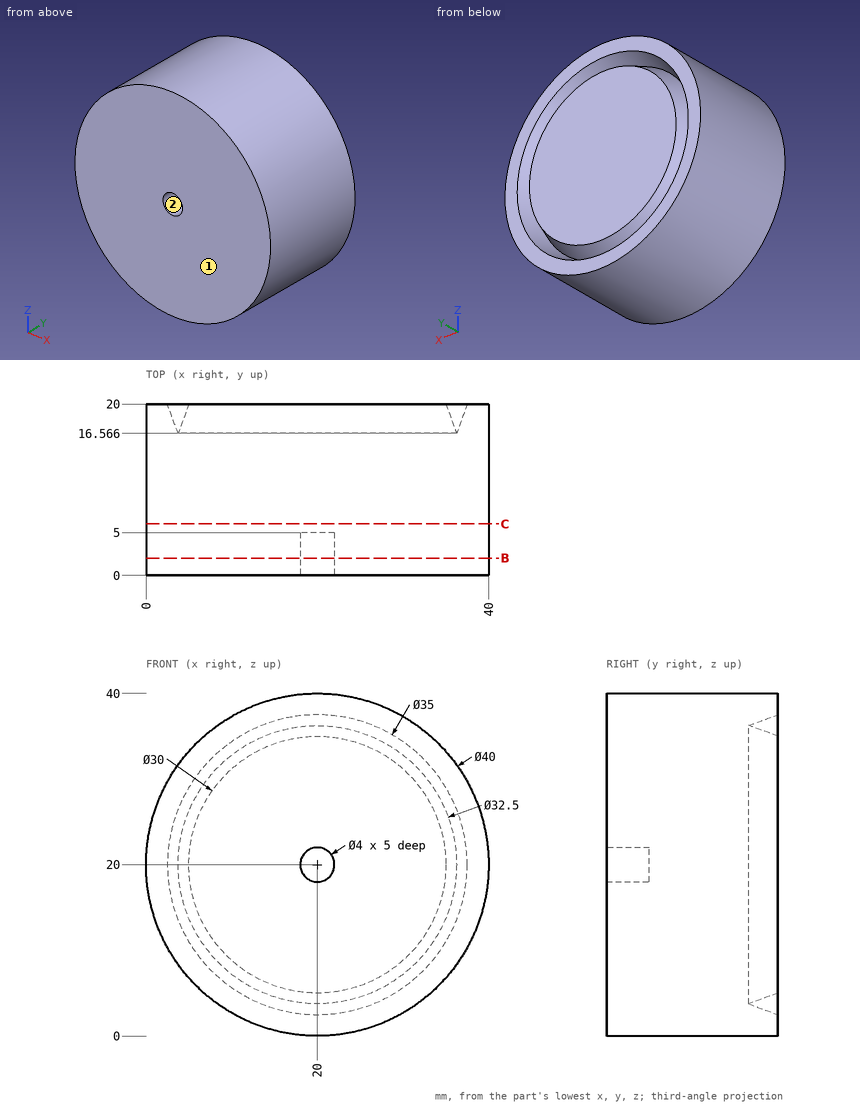
Design review of the part shown in the three views and the two pictorial views. Dimensions are in mm from the part's minimum x, y and z. A direction names the side the tool comes from. Round coordinates to 2 decimals unless told otherwise and drop trailing zeros. Loops run counter-clockwise (first coordinate to the right, second up) from the corner with the lowest first, then second, coordinate; pieces in that order, holes last. Notation, with made-up numbers: M 12,33 L 20,33 A25 ccw 20,65 Z; hole C 78.25,-13 d4. An arc over 180 degrees is marked long. Answer as a JSON object with one key per item and string values.
Item 1: Tool access review of the marked faces 1 and 2: name each direction out of +Z, -Z, +X, -X, +Y, -Y from which nothing blocks a thin tool from reaching the whole face with its end or side.
Check sheet entries:
{"face 1": "+Z, -Z, +X, -X, -Y", "face 2": "-Y"}
Item 2: For line 1 along X through (y, z) = (1.05, 20); line 2 along Z through (x, y) = (11, 19.25); line 3 along X through (y, z) = (17.25, 27.5) (1 decimal), list the stretches that pass through material, from the lowest coordinate up.
Check sheet entries:
{"line 1": "0 to 18, 22 to 40", "line 2": "2.14 to 5.31, 7.66 to 32.34, 34.69 to 37.86", "line 3": "1.5 to 5.3, 5.9 to 34.1, 34.7 to 38.5"}
Item 3: We need section C-C, the plane y = 6. State the section outline as (x, z) points.
Check sheet entries:
{"outline": "C 20,20 d40"}
Item 4: We need section B-B, the plane y = 2. State the section outline as (x, z) points, and give its area (3 significant figures).
Check sheet entries:
{"outline": "C 20,20 d40; hole C 20,20 d4", "area": "1,240 mm2"}
Item 5: Clearance check with flat-ended pins moving along their axes: P1, Ø6, axis at x = 12, y = 16, coming from the +Z side (1 decimal); P2, Ø1.5, axis at x = 4.5, y = 9, coming from the +Z side; P3, Ø1.2, axis at x = 20.5, z = 21, coming from the -Y side. State where each tip first meets the part, or that it passes through.
Check sheet entries:
{"P1": "z = 39.4", "P2": "z = 33.51", "P3": "y = 5"}
